The model under review builds one solid part; all positions refer to its coordinate system, in mm. Face numbers are marked on the shaded views. Round coordinates to 2 decimals unless told otherwise and drop trailing zeros. Write each loop counter-clockwise with the first axis right and the second up, starting at its lowest first coordinate (ties: lowest second). Pieces come first, ordered by that corner, then holes. Notation, with made-up numbers: M 33.25,81.5 L 49.25,81.5 A24 ccw 49.25,101.5 Z; hole C 58.5,-27 d6. An arc over 180 degrees is marked long. Write item = value, one per line. Start each with the question number.
Item 1: The part is to be moulded in two halves that separate along Y. For the marked faces 1, 2 and 3, say which applies: +Y half, -Y half, draft (parallel to the pull), parting line (faces both ways), or undercut.
Item 2: Take a section at A-A, the plane z = -41. Give the boundary of the cut face in (x, y).
Item 3: For pin 1 Ø12 at (x, z) = (37.5, 34.5) entering from -Y; pin 2 Ø20.5 at (x, y) = (-40.45, -4.71) entering from +Z, all flat-tipped, find the tip position at first contact; note any pin that passes through.
Item 4: To check wall thickness, follow line 1 along X through (y, z) = (-8, -9.5); line 2 along X through (y, z) = (-5, 4.5); line 3 along X through (y, z) = (-14, -35.5). State the ranges of each line that lie inside material, in increasing order.
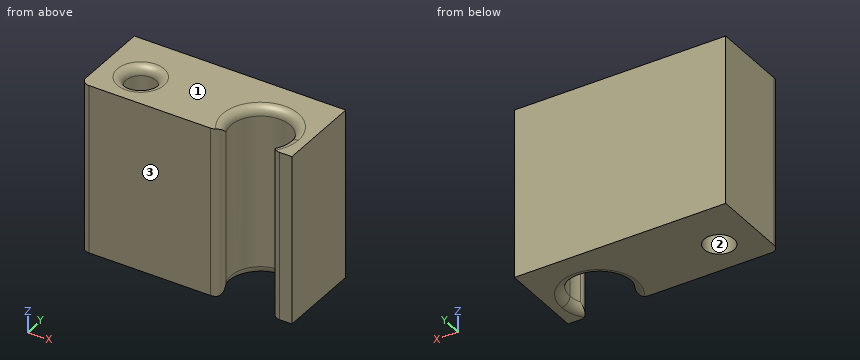
from build123d import *

# Parameters (mm, degrees)
F0_W     = 127
F0_H     = 101.6
F1_DEPTH = 25.4
F2_R     = 8.9887280552
F3_DEPTH = 101.6
F4_R     = 5.08


with BuildPart() as f1:
    # F0 (on Front) → F1 (new body, symmetric)
    with BuildSketch(Plane.XZ):
        Rectangle(F0_W, F0_H)
    extrude(amount=F1_DEPTH, both=True)

    # F2 (on face) → F3 (cut, through all)
    with BuildSketch(Plane.XY.offset(50.8)):
        with Locations((-40.4497459531, -4.7117564827)):
            Circle(F2_R)
        with BuildLine():
            ThreePointArc((45.4471273464, -25.4), (51.0720367799, -19.060106955), (53.1023527343, -10.8313970268))
            ThreePointArc((53.1023527343, -10.8313970268), (27.1833296796, 4.8286001454), (25.3769518691, -25.4))
            Line((25.3769518691, -25.4), (45.4471273464, -25.4))
        make_face()
    extrude(amount=-F3_DEPTH, mode=Mode.SUBTRACT)

    # F4
    f4_edges = [f1.edges().sort_by_distance(p)[0] for p in [
        (25.376952, -25.4, 0),
        (45.447127, -25.4, 0),
        (-63.5, -25.4, 0),
        (-49.438474, -4.711756, 50.8),
        (35.41204, 6.858916, 50.8),
        (35.41204, 6.858916, -50.8),
    ]]
    fillet(f4_edges, radius=F4_R)


solid = f1.part
Response values:
q1.face_1 = draft
q1.face_2 = undercut
q1.face_3 = -Y half
q2.outline = M -63.5,-20.32 A5.08 ccw -58.42,-25.4 L 14.71,-25.4 A5.08 ccw 19.33,-18.2 A17.69 cw long 51.49,-18.2 A5.08 ccw 56.11,-25.4 L 63.5,-25.4 L 63.5,25.4 L -63.5,25.4 Z; hole C -40.45,-4.71 d17.98
q3.pin_1 = 4.9
q3.pin_2 = 49.07
q4.line_1 = -63.5 to -48.82, -32.08 to 17.95, 52.87 to 63.5
q4.line_2 = -63.5 to -49.43, -31.47 to 18.71, 52.11 to 63.5
q4.line_3 = -63.5 to 18.01, 52.82 to 63.5
